from build123d import *

# Parameters (mm, degrees)
BOSS_EXTRUDE1_DEPTH = 19.05
SKETCH2_R           = 1.905
SKETCH2_R_2         = 4.445
SKETCH2_R_3         = 3.175
CUT_EXTRUDE1_DEPTH  = 2.54


with BuildPart() as part:
    # Sketch1 → Boss-Extrude1 (new body)
    with BuildSketch(Plane(origin=(0, 0, 0), x_dir=(1, 0, 0), z_dir=(0, 1, 0))):
        Polygon((-9.525, 48.26), (-9.525, 67.31), (-66.675, 67.31), (-66.675, 48.26), (-85.725, 48.26), (-85.725, 29.21), (-65.405, 29.21), (-65.405, 8.89), (-85.725, 8.89), (-85.725, -46.99), (-65.405, -46.99), (-65.405, -67.31), (-8.255, -67.31), (-8.255, -49.53), (9.525, -49.53), (9.525, 8.89), (-8.255, 8.89), (-8.255, 26.67), (9.525, 26.67), (9.525, 48.26), align=None)
    extrude(amount=BOSS_EXTRUDE1_DEPTH)

    # Sketch2 → Cut-Extrude1 (cut)
    with BuildSketch(Plane(origin=(0, 19.05, 0), x_dir=(1, 0, 0), z_dir=(0, 1, 0))):
        with Locations(Location((-3.175, -19.685, 0), (0, 0, 270))):
            Circle(SKETCH2_R)
        with Locations(Location((-73.025, -19.685, 0), (0, 0, 270))):
            Circle(SKETCH2_R_2)
        with Locations(Location((-38.1, 54.61, 0), (0, 0, 270))):
            Circle(SKETCH2_R_3)
    extrude(amount=-CUT_EXTRUDE1_DEPTH, mode=Mode.SUBTRACT)


solid = part.part
Can you work these out from the model? Positions are in its coordinate system, mm. A direction names the side the tool comes from. Round coordinates to 2 decimals unless told otherwise and drop trailing zeros. Loops run counter-clockwise (first coordinate to the right, second up) from the corner with the lowest first, then second, coordinate; pieces in that order, holes last. Notation, with made-up numbers: (-34, -13.75) - (-5, -13.75) arc R13 cw to (-5, 3.25) - close; hole circle Ø4 at (16.5, 75.5). An arc over 180 degrees is marked (long way). Answer in a Markdown table with one row per item. Add a question column.
Q1. I want a section at D-D on z = -13. List the corners of the cut face in (x, y) for me (3 decimals).
Q2. Which directions (+Z, -Z, +X, -X, +Y, -Y) give clear straight access to the entire face, cutting with the end or side of a thin tool? Please do faces 1 (the flat face through (0, 9, -48.26)), 2 (the flat face through (-76, 9, 46.99)), 3 (the flat face through (-8.255, 9, 59)), 4 (the flat face through (1, 9, -26.67)), 5 (the cylindrical face through (-35.954, 17.798, -56.95)).
Q3. We'd pull the mould along Z, two halves only. Please class faces 6 (the flat face through (-76, 9, -48.26)), 7 (the flat face through (-76, 9, -29.21)), 8 (the flat face through (9.525, 9, 21)), 9 (the flat face through (-65.405, 9, -19)): pulls with the +Z half, pulls with the -Z half, needs draft (parallel to the pull), parting line crosses it, or undercut.
Q4. I want a section at B-B on z = -54.61. List the corners of the cut face in (x, y) for me (3 decimals), and give its area (3 significant figures).
Q5. I want a section at C-C on y = 14.5. List the corners of the cut face in (x, z) for me (3 decimals), and give its area (3 significant figures).
Q6. I want a section at A-A on x = 3. List the corners of the cut face in (y, z) for me, and give its area (3 significant figures).
Q7. For pin 1 Ø6 at (y, z) = (8, -21.5) entering from +X (3 decimals); pin 2 Ø3.5 at (x, z) = (-3.175, 19.685) entering from +Y; pin 3 Ø5.5 at (x, y) = (-1.5, 7.5) entering from -Z, each with a flat end and sliding along its axis, tell me the tip position at first contact or that it passes through.
Q8. I need wall thicknesses on L1, parallel to X at y = 18.25, z = -54.61 (3 decimals); L2, parallel to Z at x = -79, y = 11.75; L3, parallel to Z at x = -6, y = 9.5. Which ranges of each line are inside material? Lowest first, please.
A:
| question | item | result |
|---|---|---|
| 1 | outline | (-65.405, 0) - (-8.255, 0) - (-8.255, 19.05) - (-65.405, 19.05) - close |
| 2 | face 1 | -Z, +X, +Y, -Y |
| 2 | face 2 | +Z, -X, +Y, -Y |
| 2 | face 3 | +Z, +X, +Y, -Y |
| 2 | face 4 | +X, +Y, -Y |
| 2 | face 5 | +Y |
| 3 | face 6 | pulls with the -Z half |
| 3 | face 7 | undercut |
| 3 | face 8 | needs draft |
| 3 | face 9 | undercut |
| 4 | outline | (-66.675, 0) - (-9.525, 0) - (-9.525, 19.05) - (-34.925, 19.05) - (-34.925, 16.51) - (-41.275, 16.51) - (-41.275, 19.05) - (-66.675, 19.05) - close |
| 4 | area | 1,070 mm^2 |
| 5 | outline | (-85.725, -48.26) - (-66.675, -48.26) - (-66.675, -67.31) - (-9.525, -67.31) - (-9.525, -48.26) - (9.525, -48.26) - (9.525, -26.67) - (-8.255, -26.67) - (-8.255, -8.89) - (9.525, -8.89) - (9.525, 49.53) - (-8.255, 49.53) - (-8.255, 67.31) - (-65.405, 67.31) - (-65.405, 46.99) - (-85.725, 46.99) - (-85.725, -8.89) - (-65.405, -8.89) - (-65.405, -29.21) - (-85.725, -29.21) - close |
| 5 | area | 10,600 mm^2 |
| 6 | outline | (0, -48.26) - (19.05, -48.26) - (19.05, -26.67) - (0, -26.67) - close; (0, -8.89) - (19.05, -8.89) - (19.05, 49.53) - (0, 49.53) - close |
| 6 | area | 1,520 mm^2 |
| 7 | pin 1 | x = -8.255 |
| 7 | pin 2 | y = 16.51 |
| 7 | pin 3 | z = -48.26 |
| 8 | L1 | -66.675 to -41.275, -34.925 to -9.525 |
| 8 | L2 | -48.26 to -29.21, -8.89 to 46.99 |
| 8 | L3 | -48.26 to -26.67, -8.89 to 49.53 |
